Part model, mm, in its own coordinate system. Round coordinates to 2 decimals unless told otherwise and drop trailing zeros. Write each loop counter-clockwise with the first axis right and the second up, starting at its lowest first coordinate (ties: lowest second). Pieces come first, ordered by that corner, then holes. Notation, with made-up numbers: M 80.25,22.25 L 95.25,22.25 A31 cw 95.25,53.25 Z; hole C -26,87 d7. An arc over 180 degrees is marked long. One line per question, with ' | ' between items. Start each with the question number.
1) Saw through at B-B (y = 32). List the corners of the cut face in (x, z).
2) Saw through at C-C (z = 19). List the corners of the cut face in (x, y), plus the area to 3 significant figures.
3) Drop a flat-ended pin along its axis: pin 1 Ø2 at (x, y) = (38, 14.5) entering from -Z. Give the stop position or say it passes through.
4) Wall check: probe 1 along Y at (x, z) = (30.5, 10); probe 2 along X at (y, z) = (42, 18.5); probe 3 along X at (y, z) = (35.5, 19). Give the ranges that are in metal, low to high. Write a range as [from, to].
Solid Edge part; units mm, degrees
sketch "Sketch1" plane through (0, 0, 0) normal (0, -1, 0) x (1, 0, 0)
  line L0 (-50, 25) -> (50, 25)
  line L1 (50, 25) -> (50, -25)
  line L2 (50, -25) -> (-50, -25)
  line L3 (-50, -25) -> (-50, 25)
  dimension "D1" = 50
  dimension "D2" = 50
extrude "Protrusion1" add sketch "Sketch1" against normal blind 50
chamfer "Chamfer1" distance 5 angle 45 3 edges at (50, 50, 0) (50, 25, 25) (0, 50, 25)
chamfer "Chamfer2" distance 5 angle 45 1 edges at (-50, 50, -2.5)
chamfer "Chamfer3" distance 5 distance2 15 1 edges at (-50, 0, 0) measured on face at (-32.3333, 0, -17.1667)
chamfer "Chamfer4" distance 10 distance2 20 1 edges at (2.5, 0, -25) measured on face at (34.3333, 41.1667, -25)
chamfer "Chamfer5" distance 10 distance2 20 1 edges at (0, 0, 25) measured on face at (-35.1167, 37.05, 25)
chamfer "Chamfer6" distance 10 angle 75 1 edges at (50, 27.5, -25) measured on face at (50, 37.05, 12.95)
chamfer "Chamfer7" distance 10 angle 45 2 edges at (-1.6667, 10, 25) (-50, 30, 25) measured on face at (-35.1167, 38.8167, 25)
properties material "알루미늄, 1060"
Answer key:
1) outline: M -50,-25 L 12.68,-25 L 50,-15 L 50,20 L 45,25 L -40,25 L -50,15 Z
2) outline: M -46,13.99 L 50,13.99 L 50,45 L 45,50 L -45,50 L -46,49 Z | area: 3,440 mm2
3) pin 1: stops at z = -18.48
4) probe 1: y = [4.99, 50] | probe 2: x = [-46.5, 50] | probe 3: x = [-46, 50]
